from build123d import *

# Parameters (mm, degrees)
SKETCH1_W                 = 27.99999988
SKETCH1_H                 = 28
BOSS_EXTRUDE1_DEPTH       = 3.175
SKETCH6_W                 = 27.99999988
SKETCH6_H                 = 3.175
BOSS_EXTRUDE2_DEPTH       = 38.1
CUT_EXTRUDE3_DEPTH        = 4.175
F_4_CLEARANCE_HOLE1_D     = 2.9464
F_4_CLEARANCE_HOLE1_DEPTH = 12.954
F_4_CLEARANCE_HOLE1_TIP   = 0.885187864
SKETCH10_W                = 27.99999988
SKETCH10_H                = 28.448
CUT_EXTRUDE4_DEPTH        = 4.175


with BuildPart() as part:
    # Sketch1 → Boss-Extrude1 (new body)
    with BuildSketch(Plane.XY):
        Rectangle(SKETCH1_W, SKETCH1_H)
    extrude(amount=BOSS_EXTRUDE1_DEPTH)

    # Sketch6 → Boss-Extrude2 (add)
    with BuildSketch(Plane(origin=(0, 14, 0), x_dir=(1, 0, 0), z_dir=(0, 1, 0))):
        with Locations((0, -1.5875)):
            Rectangle(SKETCH6_W, SKETCH6_H)
    extrude(amount=BOSS_EXTRUDE2_DEPTH)

    # Sketch7 → Cut-Extrude3 (cut, through all)
    with BuildSketch(Plane(origin=(0, 0, 0), x_dir=(-1, 0, 0), z_dir=(0, 0, -1))):
        with BuildLine():
            Line((-12.94999994, 45.6), (-12.94999994, 49.6))
            ThreePointArc((-12.94999994, 49.6), (-11.49999994, 51.05), (-10.04999994, 49.6))
            Line((-10.04999994, 49.6), (-10.04999994, 45.6))
            ThreePointArc((-10.04999994, 45.6), (-11.49999994, 44.15), (-12.94999994, 45.6))
        make_face()
        with BuildLine():
            Line((10.05000006, 45.6), (10.05000006, 49.6))
            ThreePointArc((10.05000006, 49.6), (11.50000006, 51.05), (12.95000006, 49.6))
            Line((12.95000006, 49.6), (12.95000006, 45.6))
            ThreePointArc((12.95000006, 45.6), (11.50000006, 44.15), (10.05000006, 45.6))
        make_face()
        with BuildLine():
            Line((-12.94999994, 22.6), (-12.94999994, 26.6))
            ThreePointArc((-12.94999994, 26.6), (-11.49999994, 28.05), (-10.04999994, 26.6))
            Line((-10.04999994, 26.6), (-10.04999994, 22.6))
            ThreePointArc((-10.04999994, 22.6), (-11.49999994, 21.15), (-12.94999994, 22.6))
        make_face()
        with BuildLine():
            Line((10.05000006, 22.6), (10.05000006, 26.6))
            ThreePointArc((10.05000006, 26.6), (11.50000006, 28.05), (12.95000006, 26.6))
            Line((12.95000006, 26.6), (12.95000006, 22.6))
            ThreePointArc((12.95000006, 22.6), (11.50000006, 21.15), (10.05000006, 22.6))
        make_face()
        with BuildLine():
            Line((-11.176, 34.1), (-11.176, 38.1))
            ThreePointArc((-11.176, 38.1), (0, 49.276), (11.176, 38.1))
            Line((11.176, 38.1), (11.176, 34.1))
            ThreePointArc((11.176, 34.1), (0, 22.924), (-11.176, 34.1))
        make_face()
    extrude(amount=-CUT_EXTRUDE3_DEPTH, mode=Mode.SUBTRACT)

    # #4 Clearance Hole1
    with Locations(Plane(origin=(0, 0, 0), x_dir=(-1, 0, 0), z_dir=(0, 0, -1))):
        with Locations((-6.35, 16.345772244), (6.35, 16.345772244)):
            Hole(F_4_CLEARANCE_HOLE1_D / 2, depth=F_4_CLEARANCE_HOLE1_DEPTH)
            with Locations((0, 0, -(F_4_CLEARANCE_HOLE1_DEPTH + F_4_CLEARANCE_HOLE1_TIP / 2))):  # 118° drill point
                Cone(0, F_4_CLEARANCE_HOLE1_D / 2, F_4_CLEARANCE_HOLE1_TIP, mode=Mode.SUBTRACT)

    # Sketch10 → Cut-Extrude4 (cut, through all)
    with BuildSketch(Plane(origin=(0, 0, 0), x_dir=(-1, 0, 0), z_dir=(0, 0, -1))):
        with Locations((0, 0.224)):
            Rectangle(SKETCH10_W, SKETCH10_H)
    extrude(amount=-CUT_EXTRUDE4_DEPTH, mode=Mode.SUBTRACT)


solid = part.part
Build history of the part. All positions in model axes, mm. A direction names the side the tool comes from. Give positions to 0.01 mm unless a question says otherwise; leave off trailing zeros. Loops run counter-clockwise (first coordinate to the right, second up) from the corner with the lowest first, then second, coordinate; pieces in that order, holes last. Notation, with made-up numbers: (53.25, 39.5) - (108.25, 39.5) arc R36 ccw to (108.25, 75.5) - close; hole circle Ø6 at (64, 79.5). An arc over 180 degrees is marked (long way). Write item = value, one per line. Start each with the question number.
1) Band-saw the part on B-B on y = 36.5. Give the cut face in (x, z) (3 decimals), plus the area to 3 significant figures.
2) Band-saw the part on D-D on x = -6.35. Give the cut face in (y, z) (3 decimals).
3) Probe probe 1 along X at (y, z) = (49.5, 2.8); probe 2 along X at (y, z) = (38.5, 0.3); probe 3 along X at (y, z) = (43, 0.7). List the from-to ranges inside material, lowest first. Write a range as from..to.
4) Tool access for faces 1 (the flat face through (-12.95, 48, 2)), 2 (the flat face through (-6.4, 24.6, 0)): list every direction of +Z, -Z, +X, -X, +Y, -Y with a clear straight run to the whole face (end or side of a thin tool).
5) Band-saw the part on C-C on z = 1.1. Give the cut face in (x, y).
6) Band-saw the part on A-A on x = 4.25. Give the cut face in (y, z) (3 decimals), plus the area to 3 significant figures.
Final values:
q1.outline = (-14, 0) - (-11.176, 0) - (-11.176, 3.175) - (-14, 3.175) - close; (11.176, 0) - (14, 0) - (14, 3.175) - (11.176, 3.175) - close
q1.area = 17.9 mm²
q2.outline = (14.448, 0) - (14.873, 0) - (14.873, 3.175) - (14.448, 3.175) - close; (17.819, 0) - (24.903, 0) - (24.903, 3.175) - (17.819, 3.175) - close; (47.297, 0) - (52.1, 0) - (52.1, 3.175) - (47.297, 3.175) - close
q3.probe_1 = -14..-12.95, -10.05..10.05, 12.95..14
q3.probe_2 = -14..-11.17, 11.17..14
q3.probe_3 = -14..-10.04, 10.04..14
q4.face_1 = +Z, -Z
q4.face_2 = -Z, +X, -X, +Y, -Y
q5.outline = (-14, 14.45) - (14, 14.45) - (14, 52.1) - (-14, 52.1) - close; hole (-12.95, 22.6) arc R1.45 ccw to (-10.05, 22.6) - (-10.05, 26.6) arc R1.45 ccw to (-12.95, 26.6) - close; hole (-12.95, 45.6) arc R1.45 ccw to (-10.05, 45.6) - (-10.05, 49.6) arc R1.45 ccw to (-12.95, 49.6) - close; hole (-11.18, 34.1) arc R11.18 ccw to (11.18, 34.1) - (11.18, 38.1) arc R11.18 ccw to (-11.18, 38.1) - close; hole circle Ø2.95 at (-6.35, 16.35); hole circle Ø2.95 at (6.35, 16.35); hole (10.05, 22.6) arc R1.45 ccw to (12.95, 22.6) - (12.95, 26.6) arc R1.45 ccw to (10.05, 26.6) - close; hole (10.05, 45.6) arc R1.45 ccw to (12.95, 45.6) - (12.95, 49.6) arc R1.45 ccw to (10.05, 49.6) - close
q6.outline = (14.448, 0) - (23.764, 0) - (23.764, 3.175) - (14.448, 3.175) - close; (48.436, 0) - (52.1, 0) - (52.1, 3.175) - (48.436, 3.175) - close
q6.area = 41.2 mm²
